Build history of the part. All positions in model axes, mm. A direction names the side the tool comes from. Coordinates: 2 decimals unless noted, no trailing zeros. Order: outer loops, then holes, each group sorted by start corner. A loop starts at its lowest first (then second) coordinate and runs counter-clockwise, first axis right, second up. Notation, with made-up numbers: M 46,74 L 75,74 A19 ccw 75,90 Z; hole C 50,87.25 d7. An arc over 180 degrees is marked long. Write item = value, one per line. Start each with the question number.
Q1. Band-saw the part on B-B on x = -7. Write the cut outline in (y, z), plus the area to 3 significant figures.
Q2. Drill centre lines: probe 1 along Z at (x, y) = (-3, -3.75); probe 2 along X at (y, z) = (-12, 4.5); probe 3 along Y at (x, z) = (-7, 4.6). Where is each one in solid material? Low to high.
Q3. Band-saw the part on C-C on z = 0. Write the cut outline in (x, y).
Q4. Pull direction X, two halves, no side cores. Call faces 1 (the face through (27, -13, 7)), 2 (the face through (13.254, -4.9, 6.5)), 3 (the face through (20.11, -0.12, -5.01)): released by +X, released by -X, zero draft, split by the parting line, or undercut.
Q5. 3-axis set-ups, long thin cutter, end or side, ignore diameter. For faces 4 (the face through (30.25, -10.23, -5.01)), 5 (the face through (-5.6, -3.8, 2.8)), 6 (the face through (-11.746, -5, -4)), 7 (the face through (26.1, -4.46, 0.59)), 8 (the face through (1, -5, 6)): which of +Z, -Z, +X, -X, +Y, -Y reach the whole face in a straight line?
Q6. Band-saw the part on D-D on y = -5. State how many separate pieces and enclosed holes the cut face has, plus the area to 3 significant figures.
Q7. Band-saw the part on A-A on x = 0. Write the cut outline in (y, z), plus the area to 3 significant figures.
Q8. Pin check, flat tips, straight feed: P1, Ø3.5, axis at x = -7, y = -5, coming from the +Z side; P2, Ø5, axis at y = -15, z = 5.5, coming from the -X side; P3, Ø1, axis at x = 5.5, z = -3, coming from the +Y side. Stop position of each tip, or through.
```python
from build123d import *

# Parameters (mm, degrees)
PAD_DEPTH            = 10
SKETCH_R             = 1.6
PAD001_DEPTH         = 7
PAD001_DEPTH_BACK    = 6
SKETCH004_R          = 3
POCKET_DEPTH         = 27.372693
POCKET001_DEPTH      = 2
SKETCH006_R          = 1.6
POCKET002_DEPTH      = 6.001
POCKET002_DEPTH_BACK = -7.001


with BuildPart() as part:
    # Sketch003 → Pad (new body)
    with BuildSketch(Plane.XZ):
        with BuildLine():
            Line((13.253575, -6), (-11.746425, -6))
            Line((-11.746425, -2.8), (-11.746425, -6))
            Line((-1.746425, -2.8), (-11.746425, -2.8))
            ThreePointArc((-1.746425, -2.8), (3.3, 0), (-1.746425, 2.8))
            Line((-1.746425, 2.8), (-11.746425, 2.8))
            Line((-11.746425, 2.8), (-11.746425, 6))
            Line((13.253575, 6), (-11.746425, 6))
            Line((13.253575, 6), (13.253575, 0))
            Line((13.253575, 0), (13.253575, -6))
        make_face()
    extrude(amount=PAD_DEPTH)

    # Sketch → Pad001 (join, two sides)
    with BuildSketch(Plane.XY) as pad001_sk:
        Polygon((13.253575, -10), (20.324643, -17.071068), (30.324643, -17.071068), (34.517031, -12.87868), (17.445963, 4.192388), (13.253575, 0), align=None)
        with Locations((17.445963, -0.807612)):
            Circle(SKETCH_R, mode=Mode.SUBTRACT)
        with Locations((29.517031, -12.87868)):
            Circle(SKETCH_R, mode=Mode.SUBTRACT)
    extrude(amount=PAD001_DEPTH)
    extrude(pad001_sk.sketch, amount=-PAD001_DEPTH_BACK)

    # Sketch004 (on DatumPlane) → Pocket (cut, through all)
    with BuildSketch(Plane(origin=(0, 0, 3.5), x_dir=(0, 0, -1), z_dir=(-0.707107, -0.707107, 0))):
        with Locations((-3.5, 21.442761)):
            Circle(SKETCH004_R)
    extrude(amount=-POCKET_DEPTH, mode=Mode.SUBTRACT)

    # Sketch005 (on DatumPlane) → Pocket001 (cut)
    with BuildSketch(Plane.XY.offset(-6)):
        Polygon((18.267824, -3.874838), (20.51319, -1.629473), (19.691329, 1.437754), (16.624102, 2.259615), (14.378737, 0.014249), (15.200598, -3.052977), align=None)
        Polygon((30.338892, -15.945906), (32.584257, -13.700541), (31.762397, -10.633314), (28.69517, -9.811453), (26.449805, -12.056819), (27.271665, -15.124045), align=None)
    extrude(amount=POCKET001_DEPTH, mode=Mode.SUBTRACT)

    # Sketch006 → Pocket002 (cut, two sides)
    with BuildSketch(Plane.XY) as pocket002_sk:
        with Locations((-7, -5)):
            Circle(SKETCH006_R)
    extrude(amount=-POCKET002_DEPTH, mode=Mode.SUBTRACT)
    extrude(pocket002_sk.sketch, amount=-POCKET002_DEPTH_BACK, mode=Mode.SUBTRACT)


solid = part.part
```
Recorded:
q1.outline = M -10,-6 L -6.6,-6 L -6.6,-2.8 L -10,-2.8 Z; M -10,2.8 L -6.6,2.8 L -6.6,6 L -10,6 Z; M -3.4,-6 L 0,-6 L 0,-2.8 L -3.4,-2.8 Z; M -3.4,2.8 L 0,2.8 L 0,6 L -3.4,6 Z
q1.area = 43.5 mm2
q2.probe_1 = -6 to -2.8, 2.8 to 6
q2.probe_2 = 15.25 to 15.98, 20.67 to 28.18, 30.85 to 33.64
q2.probe_3 = -10 to -6.6, -3.4 to 0
q3.outline = M 3.3,-10 L 13.25,-10 L 20.32,-17.07 L 30.32,-17.07 L 34.52,-12.88 L 17.45,4.19 L 13.25,0 L 3.3,0 Z; hole C 17.45,-0.81 d3.2; hole C 29.52,-12.88 d3.2
q4.face_1 = zero draft
q4.face_2 = released by -X
q4.face_3 = undercut
q5.face_4 = -Z
q5.face_5 = -X, +Y, -Y
q5.face_6 = +Z, -Z, -X, +Y, -Y
q5.face_7 = +Z, -Z, +X, +Y
q5.face_8 = +Z, -X, +Y, -Y
q6.separate_pieces = 3
q6.enclosed_holes = 0
q6.area = 356 mm2
q7.outline = M -10,-6 L 0,-6 L 0,-3.3 L -10,-3.3 Z; M -10,3.3 L 0,3.3 L 0,6 L -10,6 Z
q7.area = 54.0 mm2
q8.P1 = 6
q8.P2 = 16.16
q8.P3 = 0
